Input: part model. Units: mm. Frame: model coordinates. A direction names the side the tool comes from. Round coordinates to 2 decimals unless told otherwise and drop trailing zeros. Loops run counter-clockwise (first coordinate to the right, second up) from the corner with the lowest first, then second, coordinate; pieces in that order, holes last.
1) Section B-B, the plane z = -64. Return loops of the section in (x, y).
2) Access query for faces 1 (the face through (-92, 98.125, -45)), 2 (the face through (-166, 93, -6.055)), 3 (the face through (-64, 10, 66)), 4 (the face through (-92, 88.08, -45)). Directions: +Z, -Z, +X, -X, +Y, -Y. A direction counts if a zero-diameter tool reaches every point of the face in a straight line with its end or side. Return the directions, or none.
3) Section A-A, the plane y = 91. Return loops of the section in (x, z).
4) First-contact query: pin 1 (5 mm diameter, centred on x = -63, y = 72, fed in from -Z); pin 2 (8 mm diameter, centred on x = -179, y = 91, fed in from +Z); pin 3 (11 mm diameter, centred on y = 95, z = -62, fed in from +X). Flat tips, straight axial feed; report the tip coordinate or a pass-through.
5) Draft query along X for faces 5 (the face through (-196.443, 93, -45)), 6 (the face through (-63, 49, 143.945)), 7 (the face through (-64, 56, 137.296)). Return one class per face: pulls with the +X half, pulls with the -X half, needs draft (parallel to the pull), parting line crosses it, or undercut.
6) Section C-C, the plane x = -160. Return loops of the section in (y, z).
7) Section D-D, the plane y = 63. Return loops of the section in (x, z).
8) Ray query, line 1 along X through (y, z) = (77, 64.5); line 2 along Z through (x, y) = (-176, 96.5); line 3 along Z through (x, y) = (-129.5, 23). Return the intervals inside material, ascending.
from build123d import *

# Parameters (mm, degrees)
SKETCH_1_W          = 150
SKETCH_1_H          = 150
EXTRUDE_1_DEPTH     = 100
SKETCH_2_W          = 140
SKETCH_2_H          = 140
CUT_EXTRUDE_1_DEPTH = 90
SKETCH_3_W          = 206.584523794
SKETCH_3_H          = 10.04468641
EXTRUDE_2_DEPTH     = 80
SKETCH_4_W          = 40
SKETCH_4_H          = 20
CUT_EXTRUDE_2_DEPTH = 20


with BuildPart() as part:
    # 草图1 → 凸台-拉伸1 (new body)
    with BuildSketch(Plane(origin=(0, 0, 0), x_dir=(1, 0, 0), z_dir=(0, 1, 0))):
        with Locations((-61.989619377, -68.944636678)):
            Rectangle(SKETCH_1_W, SKETCH_1_H)
    extrude(amount=EXTRUDE_1_DEPTH)

    # 草图2 → 切除-拉伸1 (cut)
    with BuildSketch(Plane(origin=(0, 100, 0), x_dir=(1, 0, 0), z_dir=(0, 1, 0))):
        with Locations((-62.547413878, -67.29555388)):
            Rectangle(SKETCH_2_W, SKETCH_2_H)
    extrude(amount=-CUT_EXTRUDE_1_DEPTH, mode=Mode.SUBTRACT)

    # 草图3 → 凸台-拉伸2 (add)
    with BuildSketch(Plane(origin=(0, 0, -6.055363322), x_dir=(-1, 0, 0), z_dir=(0, 0, -1))):
        with Locations((93.150620362, 93.10231994)):
            Rectangle(SKETCH_3_W, SKETCH_3_H)
    extrude(amount=EXTRUDE_2_DEPTH)

    # 草图4 → 切除-拉伸2 (cut)
    with BuildSketch(Plane.XZ.offset(-88.079976735)):
        with Locations((-172.313011016, -70.712776271)):
            Rectangle(SKETCH_4_W, SKETCH_4_H)
    extrude(amount=-CUT_EXTRUDE_2_DEPTH, mode=Mode.SUBTRACT)


solid = part.part
Final values:
1. outline: (-196.44, 88.08) - (-192.31, 88.08) - (-192.31, 98.12) - (-196.44, 98.12) - close; (-152.31, 88.08) - (10.14, 88.08) - (10.14, 98.12) - (-152.31, 98.12) - close
2. face 1: -Z, +X, -X, +Y
2. face 2: +Z, -X, +Y, -Y
2. face 3: +Y
2. face 4: -Z, +X, -X, -Y
3. outline: (-196.44, -86.06) - (10.14, -86.06) - (10.14, -6.06) - (13.01, -6.06) - (13.01, 143.94) - (-136.99, 143.94) - (-136.99, -6.06) - (-196.44, -6.06) - close; hole (-192.31, -80.71) - (-152.31, -80.71) - (-152.31, -60.71) - (-192.31, -60.71) - close; hole (-132.55, -2.7) - (7.45, -2.7) - (7.45, 137.3) - (-132.55, 137.3) - close
4. pin 1: stops at z = -6.06
4. pin 2: stops at z = -6.06
4. pin 3: stops at x = 10.14
5. face 5: pulls with the -X half
5. face 6: needs draft
5. face 7: undercut
6. outline: (88.08, -86.06) - (98.12, -86.06) - (98.12, -80.71) - (88.08, -80.71) - close; (88.08, -60.71) - (98.12, -60.71) - (98.12, -6.06) - (88.08, -6.06) - close
7. outline: (-136.99, -6.06) - (13.01, -6.06) - (13.01, 143.94) - (-136.99, 143.94) - close; hole (-132.55, -2.7) - (7.45, -2.7) - (7.45, 137.3) - (-132.55, 137.3) - close
8. line 1: x = -136.99 to -132.55, 7.45 to 13.01
8. line 2: z = -86.06 to -80.71, -60.71 to -6.06
8. line 3: z = -6.06 to -2.7, 137.3 to 143.94
